For this review, take the finished solid that the model builds, in its own axes (mm). Face numbers are marked on the shaded views. A direction names the side the tool comes from. Give positions to 0.01 mm unless a question says otherwise; leave off trailing zeros. Order: outer loops, then holes, each group sorted by start corner. A loop starts at its lowest first (then second) coordinate and runs counter-clockwise, first axis right, second up. Notation, with made-up numbers: (47.25, 30.25) -> (83.25, 30.25) arc R12 cw to (83.25, 53.25) -> close; hole circle Ø7 at (5, 58). An arc over 180 degrees is marked (long way). Return JSON: item names as keys, results as strings. Group by question number.
1) To check wall thickness, follow line 1 along Z through (x, y) = (-10, -5.5) (3 decimals); line 2 along X through (y, z) = (0, 10.5) (3 decimals); line 3 along Y through (x, z) = (0, 8.5). State the ranges of each line that lie inside material, in increasing order.
2) Add section D-D (z = 7). Give the boundary of the cut face in (x, y).
3) The part is to be moulded in two halves that separate along Z. For the marked faces 3, 4 and 5, say which applies: released by +Z, released by -Z, zero draft, split by the parting line, or undercut.
4) Add section A-A (y = 0). Give the boundary of the cut face in (x, z) (3 decimals).
5) Insertion check: P1, Ø8, axis at y = -5.5, z = 4.5, coming from the +X side; P2, Ø6, axis at x = 6.5, z = 4.5, coming from the +Y side; P3, Ø1, axis at x = -2, z = 3, coming from the -Y side. Each pin has a flat end and moves straight along its axis. Give the tip position at first contact, or say it passes through.
6) For the marked faces 1 and 2, list the 3-axis set-ups (+Z, -Z, +X, -X, +Y, -Y) from which the entire face can be reached by the end or side of a thin tool; tool diameter is ignored.
7) Add section B-B (x = -10.5). Give the boundary of the cut face in (y, z) (3 decimals).
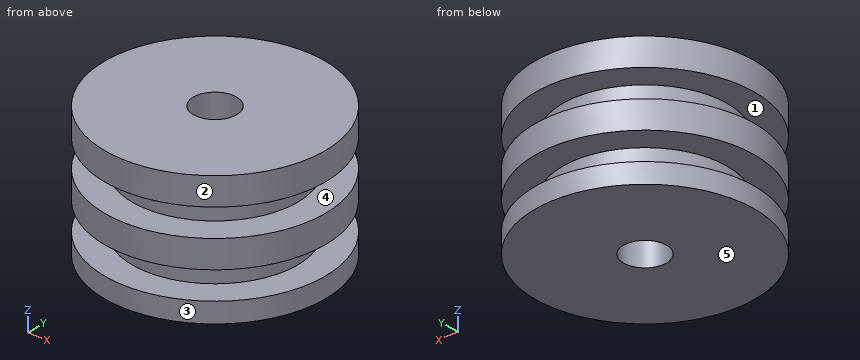
from build123d import *

# Parameters (mm, degrees)
F0_R     = 12.7
F0_R_2   = 9.525
F1_DEPTH = 15
F3_W     = 3.175
F3_H     = 3.175
F5_R     = 2.5
F6_DEPTH = 25.4


with BuildPart() as f1:
    # F0 (on Top) → F1 (new body)
    with BuildSketch(Plane.XY):
        Circle(F0_R)
        Circle(F0_R_2, mode=Mode.SUBTRACT)
        Circle(F0_R_2)
    extrude(amount=F1_DEPTH)

    # F3 (on Right) → F4 (revolve, cut)
    with BuildSketch(Plane.YZ):
        with Locations((11.1125, 3.8875)):
            Rectangle(F3_W, F3_H)
        with Locations((11.1125, 10.2375)):
            Rectangle(F3_W, F3_H)
    revolve(axis=Axis((0, 0, -0.284396), (0, 0, 1)), mode=Mode.SUBTRACT)

    # F5 (on face) → F6 (cut)
    with BuildSketch(Plane.XY):
        Circle(F5_R)
    extrude(amount=F6_DEPTH, mode=Mode.SUBTRACT)


solid = f1.part
Evaluation:
{
 "1": {"line 1": "0 to 2.3, 5.475 to 8.65, 11.825 to 15", "line 2": "-9.525 to -2.5, 2.5 to 9.525", "line 3": "-12.7 to -2.5, 2.5 to 12.7"},
 "2": {"outline": "circle Ø25.4 at (0, 0); hole circle Ø5 at (0, 0)"},
 "3": {"face 3": "zero draft", "face 4": "undercut", "face 5": "released by -Z"},
 "4": {"outline": "(-12.7, 0) -> (-2.5, 0) -> (-2.5, 15) -> (-12.7, 15) -> (-12.7, 11.825) -> (-9.525, 11.825) -> (-9.525, 8.65) -> (-12.7, 8.65) -> (-12.7, 5.475) -> (-9.525, 5.475) -> (-9.525, 2.3) -> (-12.7, 2.3) -> close; (2.5, 0) -> (12.7, 0) -> (12.7, 2.3) -> (9.525, 2.3) -> (9.525, 5.475) -> (12.7, 5.475) -> (12.7, 8.65) -> (9.525, 8.65) -> (9.525, 11.825) -> (12.7, 11.825) -> (12.7, 15) -> (2.5, 15) -> close"},
 "5": {"P1": "x = 12.6", "P2": "y = 12.16", "P3": "y = -9.41"},
 "6": {"face 1": "none", "face 2": "+Z, -Z"},
 "7": {"outline": "(-7.144, 0) -> (7.144, 0) -> (7.144, 2.3) -> (-7.144, 2.3) -> close; (-7.144, 5.475) -> (7.144, 5.475) -> (7.144, 8.65) -> (-7.144, 8.65) -> close; (-7.144, 11.825) -> (7.144, 11.825) -> (7.144, 15) -> (-7.144, 15) -> close"}
}
